Source: CAD feature listing. Evaluate the final solid. Frame: model axes, mm. A direction names the side the tool comes from. Give positions to 0.01 mm unless a question says otherwise; leave off trailing zeros. Loops run counter-clockwise (first coordinate to the right, second up) from the corner with the lowest first, then second, coordinate; pieces in that order, holes last. Notation, with made-up numbers: M 50,68.25 L 73,68.25 A21 cw 73,82.25 Z; hole C -16,20.5 d6. An arc over 180 degrees is marked long. Answer in a Markdown table with one row per item.
```python
from build123d import *

# Parameters (mm, degrees)
BOSS_EXTRUDE1_DEPTH = 5.5
FILLET1_R           = 5.5
SKETCH2_R           = 3.5
CUT_EXTRUDE1_DEPTH  = 79.760713557
SKETCH3_W           = 16
SKETCH3_H           = 5
BOSS_EXTRUDE2_DEPTH = 8
SKETCH4_R           = 1.75
CUT_EXTRUDE2_DEPTH  = 70.571905249
CHAMFER1_SIZE       = 6


# Some blends are built 0.0001 mm under size
with BuildPart() as part:
    # Sketch1 → Boss-Extrude1 (new, symmetric)
    with BuildSketch(Plane(origin=(0, 0, 0), x_dir=(1, 0, 0), z_dir=(0, 1, 0))):
        with BuildLine():
            Line((-16, 9), (-16, 14))
            Line((-16, 14), (0, 14))
            Line((0, 14), (11.907049388, 23.177264019))
            ThreePointArc((11.907049388, 23.177264019), (19.971251264, 27.504371267), (29, 29))
            Line((29, 29), (53, 29))
            Line((53, 29), (53, 25))
            Line((53, 25), (29, 25))
            ThreePointArc((29, 25), (12.029437252, 17.970562748), (5, 1))
            Line((5, 1), (5, -1))
            ThreePointArc((5, -1), (12.029437252, -17.970562748), (29, -25))
            Line((29, -25), (53, -25))
            Line((53, -25), (53, -29))
            Line((53, -29), (29, -29))
            ThreePointArc((29, -29), (19.971251264, -27.504371267), (11.907049388, -23.177264019))
            Line((11.907049388, -23.177264019), (0, -14))
            Line((0, -14), (-16, -14))
            Line((-16, -14), (-16, -9))
            Line((-16, -9), (0, -9))
            Line((0, -9), (0, 9))
            Line((0, 9), (-16, 9))
        make_face()
    extrude(amount=BOSS_EXTRUDE1_DEPTH, both=True)

    # Fillet1
    fillet1_edges = [part.edges().sort_by_distance(p)[0] for p in [
        (53, -5.5, 27),
        (53, 5.5, 27),
        (53, -5.5, -27),
        (53, 5.5, -27),
    ]]
    fillet(fillet1_edges, radius=FILLET1_R - 0.0001)  # a hair under: the kernel refuses the full size

    # Sketch2 → Cut-Extrude1 (cut, through all)
    with BuildSketch(Plane.XY.offset(29)):
        with Locations((47.5, 0)):
            Circle(SKETCH2_R)
    extrude(amount=-CUT_EXTRUDE1_DEPTH, mode=Mode.SUBTRACT)

    # Sketch3 → Boss-Extrude2 (add)
    with BuildSketch(Plane(origin=(0, 5.5, 0), x_dir=(1, 0, 0), z_dir=(0, 1, 0))):
        with Locations((-8, 11.5)):
            Rectangle(SKETCH3_W, SKETCH3_H)
        with Locations((-8, -11.5)):
            Rectangle(SKETCH3_W, SKETCH3_H)
    extrude(amount=BOSS_EXTRUDE2_DEPTH)

    # Sketch4 → Cut-Extrude2 (cut, through all)
    with BuildSketch(Plane.XY.offset(14)):
        with Locations((-11, 9)):
            Circle(SKETCH4_R)
        with Locations((-11, -1)):
            Circle(SKETCH4_R)
    extrude(amount=-CUT_EXTRUDE2_DEPTH, mode=Mode.SUBTRACT)

    # Chamfer1
    # the kernel refuses this chamfer: 6 mm, written as the material it adds along each edge
    with BuildSketch(Plane(origin=(0, 5.5, -29.430097928), x_dir=(0.9996219169112968, -0.027495876610586348, 0), z_dir=(0, 0, 1))) as chamfer1_piece_1_section:
        Polygon((CHAMFER1_SIZE * 0.999621916911, CHAMFER1_SIZE * 0.0274958766106), (-CHAMFER1_SIZE * 0.0274958766106, CHAMFER1_SIZE * 0.999621916911), (0, 0), align=None)
    chamfer1_piece_1 = extrude(amount=20.430097928, mode=Mode.PRIVATE)
    chamfer1_piece_1 = split(chamfer1_piece_1, bisect_by=Plane(origin=(4.348037064, 5.828125, -17.351215133), z_dir=(0.6104625218625276, 0, 0.7920451435374395)), keep=Keep.TOP, mode=Mode.PRIVATE)
    add(chamfer1_piece_1)
    with BuildSketch(Plane(origin=(0, 5.5, 9), x_dir=(0.9996219169112968, -0.027495876610586348, 0), z_dir=(0, 0, 1))) as chamfer1_piece_2_section:
        Polygon((CHAMFER1_SIZE * 0.999621916911, CHAMFER1_SIZE * 0.0274958766106), (-CHAMFER1_SIZE * 0.0274958766106, CHAMFER1_SIZE * 0.999621916911), (0, 0), align=None)
    chamfer1_piece_2 = extrude(amount=20.430097928, mode=Mode.PRIVATE)
    chamfer1_piece_2 = split(chamfer1_piece_2, bisect_by=Plane(origin=(-0.01385991, 7.547619048, 13.989317584), z_dir=(0.6104625218625275, 0, -0.7920451435374395)), keep=Keep.TOP, mode=Mode.PRIVATE)
    add(chamfer1_piece_2)


solid = part.part
```
1) Section D-D, the plane y = 12.5. Return loops of the section in (x, z), then the cut area to 3 significant figures.
Reply:
| item | result |
|---|---|
| outline | M -16,-14 L 0,-14 L 0,-9 L -16,-9 Z; M -16,9 L 0,9 L 0,14 L -16,14 Z |
| area | 160 mm² |
2) Section B-B, the plane y = 2.25. Return loops of the section in (x, z).
Reply:
| item | result |
|---|---|
| outline | M -16,-14 L 0,-14 L 11.91,-23.18 A28 ccw 29,-29 L 44.82,-29 L 44.82,-25 L 29,-25 A24 cw 5,-1 L 5,1 A24 cw 29,25 L 44.82,25 L 44.82,29 L 29,29 A28 ccw 11.91,23.18 L 0,14 L -16,14 L -16,9 L 0,9 L 0,-9 L -16,-9 Z; M 50.18,-29 L 52.52,-29 L 52.52,-25 L 50.18,-25 Z; M 50.18,25 L 52.52,25 L 52.52,29 L 50.18,29 Z |
3) Material intervals for L1, parallel to Y at x = -11, z = 11.05; L2, parallel to Z at x = -0.5, y = -4.25; L3, parallel to Z at x = 36, y = -4, sorted ascending.
Reply:
| item | result |
|---|---|
| L1 | y = -5.5 to -2.75, 0.75 to 7.25, 10.75 to 13.5 |
| L2 | z = -14 to -9, 9 to 14 |
| L3 | z = -29 to -25, 25 to 29 |
4) Pin query (flat end, axial travel): pin 1 Ø4 at (x, y) = (26.5, 3.5) entering from -Z; pin 2 Ø1 at (y, z) = (3, -6) entering from +X; pin 3 Ø5.5 at (x, y) = (-8.5, 3) entering from -Z. Return the tip coordinate at first contact, or that it passes through.
Reply:
| item | result |
|---|---|
| pin 1 | stops at z = -29 |
| pin 2 | stops at x = 5.64 |
| pin 3 | stops at z = -14 |
5) Set-up query: faces 4 (the cylindrical face through (20.093, 0.077, 27.546)), 5 (the flat face through (0, 12, -11)), 6 (the cylindrical face through (11.84, 0.08, 17.78)). Return all of +Z, -Z, +X, -X, +Y, -Y with unobstructed straight access to the full face (end or side cutting, diameter ignored); none if empty.
Reply:
| item | result |
|---|---|
| face 4 | +Z, -X, +Y, -Y |
| face 5 | +Z, -Z, +X, +Y |
| face 6 | +X, +Y, -Y |
6) Pull-direction query (X, two-part tool) for faces 1 (the flat face through (0, 0, 0)), 2 (the cylindrical face through (44, 0, -27)), 3 (the flat face through (3, 8.5, -12.8)); classes: released by +X, released by -X, zero draft, split by the parting line, or undercut.
Reply:
| item | result |
|---|---|
| face 1 | released by -X |
| face 2 | undercut |
| face 3 | released by +X |
7) Section C-C, the plane x = -11. Return loops of the section in (y, z).
Reply:
| item | result |
|---|---|
| outline | M -5.5,-14 L -2.75,-14 L -2.75,-9 L -5.5,-9 Z; M -5.5,9 L -2.75,9 L -2.75,14 L -5.5,14 Z; M 0.75,-14 L 7.25,-14 L 7.25,-9 L 0.75,-9 Z; M 0.75,9 L 7.25,9 L 7.25,14 L 0.75,14 Z; M 10.75,-14 L 13.5,-14 L 13.5,-9 L 10.75,-9 Z; M 10.75,9 L 13.5,9 L 13.5,14 L 10.75,14 Z |
8) Section A-A, the plane x = 30. Return loops of the section in (y, z), then the cut area to 3 significant figures.
Reply:
| item | result |
|---|---|
| outline | M -5.5,-29 L 5.5,-29 L 5.5,-25 L -5.5,-25 Z; M -5.5,25 L 5.5,25 L 5.5,29 L -5.5,29 Z |
| area | 88.0 mm² |
